Build history of the part. All positions in model axes, mm. A direction names the side the tool comes from. Coordinates: 2 decimals unless noted, no trailing zeros. Order: outer loops, then holes, each group sorted by start corner. A loop starts at its lowest first (then second) coordinate and runs counter-clockwise, first axis right, second up. Notation, with made-up numbers: M 51.5,-27.5 L 67.5,-27.5 A26 ccw 67.5,9.5 Z; hole C 35,-19.75 d8. An arc over 180 degrees is marked long. Write item = value, one per line. Start each with the question number.
Q1. Band-saw the part on B-B on x = 44.9. Write the cut outline in (y, z) (3 decimals).
Q2. 3-axis set-ups, long thin cutter, end or side, ignore diameter. For faces 4 (the face through (-47.285, 17.465, -14.711)), 5 (the face through (38, 15, -19)): which of +Z, -Z, +X, -X, +Y, -Y reach the whole face in a straight line?
Q3. Drill centre lines: probe 1 along X at (y, z) = (18.15, -13.73) (3 decimals); probe 2 along Y at (x, z) = (-82.5, -0.6) (1 decimal); probe 3 along X at (y, z) = (16, -13). Where is each one in solid material? Low to high.
Q4. Pin check, flat tips, straight feed: P1, Ø0.5, axis at y = 17.5, z = -21.5, coming from the +X side; P2, Ø7, axis at x = -32.5, z = -24.97, coming from the -Y side; P3, Ø3.5, axis at x = -82.5, y = -11, coming from the +Z side (3 decimals); P4, Ø1.1, axis at y = 17.5, z = -25.5, coming from the -X side. Stop position of each tip, or through.
Q5. Band-saw the part on C-C on z = -24.97. Write the cut outline in (x, y) (3 decimals).
Q6. Band-saw the part on A-A on y = -11. Write the cut outline in (x, z) (3 decimals).
Q7. Pull direction Z, two halves, no side cores. Call faces 1 (the face through (1, 1, -2.5)), 2 (the face through (96.5, 2, 0)), 3 (the face through (44.993, 17.465, -22.847)): released by +Z, released by -Z, zero draft, split by the parting line, or undercut.
Q8. Band-saw the part on D-D on x = -38.5. Write the cut outline in (y, z).
```python
from build123d import *

# Parameters (mm, degrees)
SKETCH1_W           = 193
SKETCH1_H           = 5
BOSS_EXTRUDE1_DEPTH = 15
BOSS_EXTRUDE2_DEPTH = 5
CUT_EXTRUDE1_REACH  = 109.344
SKETCH3_R           = 2.125
FILLET3_R           = 2
FILLET4_R           = 2
SKETCH4_R           = 2.125
CUT_EXTRUDE2_DEPTH  = 106.877004204


with BuildPart() as part:
    # Sketch1 → Boss-Extrude1 (new, symmetric)
    with BuildSketch(Plane(origin=(0, 0, 0), x_dir=(1, 0, 0), z_dir=(0, 1, 0))):
        Rectangle(SKETCH1_W, SKETCH1_H)
    extrude(amount=BOSS_EXTRUDE1_DEPTH, both=True)

    # Sketch2 → Boss-Extrude2 (add)
    with BuildSketch(Plane(origin=(0, 15, 0), x_dir=(1, 0, 0), z_dir=(0, 1, 0))):
        Polygon((-58.3, 36.2), (-58.3, 2.5), (-96.5, 2.5), (-96.5, -2.5), (96.5, -2.5), (96.5, 2.5), (57.8, 2.5), (57.8, 36.2), (19.1, 36.2), (19.1, 2.5), (-19.6, 2.5), (-19.6, 36.2), align=None)
    extrude(amount=BOSS_EXTRUDE2_DEPTH)

    # Sketch3 → Cut-Extrude1 (cut, up to next)
    with BuildSketch(Plane.XZ.offset(-15), mode=Mode.PRIVATE) as cut_extrude1_sk1:
        with Locations(Location((-45.4, -13.73, 0), (0, 0, 270))):
            Circle(SKETCH3_R)
    cut_extrude1_tool1 = extrude(cut_extrude1_sk1.sketch, amount=-CUT_EXTRUDE1_REACH, mode=Mode.PRIVATE) & part.part
    # Sketch3 → Cut-Extrude1 (cut, up to next)
    with BuildSketch(Plane.XZ.offset(-15), mode=Mode.PRIVATE) as cut_extrude1_sk2:
        with Locations(Location((-32.5, -24.97, 0), (0, 0, 270))):
            Circle(SKETCH3_R)
    cut_extrude1_tool2 = extrude(cut_extrude1_sk2.sketch, amount=-CUT_EXTRUDE1_REACH, mode=Mode.PRIVATE) & part.part
    # Sketch3 → Cut-Extrude1 (cut, up to next)
    with BuildSketch(Plane.XZ.offset(-15), mode=Mode.PRIVATE) as cut_extrude1_sk3:
        with Locations(Location((32, -13.73, 0), (0, 0, 270))):
            Circle(SKETCH3_R)
    cut_extrude1_tool3 = extrude(cut_extrude1_sk3.sketch, amount=-CUT_EXTRUDE1_REACH, mode=Mode.PRIVATE) & part.part
    # Sketch3 → Cut-Extrude1 (cut, up to next)
    with BuildSketch(Plane.XZ.offset(-15), mode=Mode.PRIVATE) as cut_extrude1_sk4:
        with Locations(Location((44.9, -24.97, 0), (0, 0, 270))):
            Circle(SKETCH3_R)
    cut_extrude1_tool4 = extrude(cut_extrude1_sk4.sketch, amount=-CUT_EXTRUDE1_REACH, mode=Mode.PRIVATE) & part.part
    add(cut_extrude1_tool1.solids().sort_by_distance((-45.4, 15, -13.73))[0], mode=Mode.SUBTRACT)
    add(cut_extrude1_tool2.solids().sort_by_distance((-32.5, 15, -24.97))[0], mode=Mode.SUBTRACT)
    add(cut_extrude1_tool3.solids().sort_by_distance((32, 15, -13.73))[0], mode=Mode.SUBTRACT)
    add(cut_extrude1_tool4.solids().sort_by_distance((44.9, 15, -24.97))[0], mode=Mode.SUBTRACT)

    # Fillet3
    fillet3_edges = [part.edges().sort_by_distance(p)[0] for p in [
        (-58.3, 17.5, -36.2),
        (-58.3, 17.5, -2.5),
        (57.8, 17.5, -2.5),
        (57.8, 17.5, -36.2),
        (19.1, 17.5, -36.2),
        (19.1, 17.5, -2.5),
        (-19.6, 17.5, -2.5),
        (-19.6, 17.5, -36.2),
    ]]
    fillet(fillet3_edges, radius=FILLET3_R)

    # Fillet4
    # the kernel refuses this fillet: 2 mm, written as the material it takes off along each edge
    with BuildSketch(Plane(origin=(21.1, 20, -34.2), x_dir=(-1, 0, 0), z_dir=(0, 0, 1))) as fillet4_piece_1:
        with BuildLine():
            CenterArc((2 - FILLET4_R, FILLET4_R), FILLET4_R, 270, 90)
            Line((2 - FILLET4_R, 0), (2, 0))
            Line((2, 0), (2, FILLET4_R))
        make_face()
    revolve(axis=Axis((21.1, 20, -34.2), (0, -1, 0)), revolution_arc=90, mode=Mode.SUBTRACT)
    with BuildSketch(Plane(origin=(-21.6, 20, -34.2), x_dir=(1, 0, 0), z_dir=(0, 0, 1))) as fillet4_piece_2:
        with BuildLine():
            CenterArc((2 - FILLET4_R, -FILLET4_R), FILLET4_R, 0, 90)
            Line((2 - FILLET4_R, 0), (2, 0))
            Line((2, 0), (2, -FILLET4_R))
        make_face()
    revolve(axis=Axis((-21.6, 20, -34.2), (0, 1, 0)), revolution_arc=90, mode=Mode.SUBTRACT)
    with BuildSketch(Plane(origin=(-56.3, 20, -34.2), x_dir=(-1, 0, 0), z_dir=(0, 0, 1))) as fillet4_piece_3:
        with BuildLine():
            CenterArc((2 - FILLET4_R, FILLET4_R), FILLET4_R, 270, 90)
            Line((2 - FILLET4_R, 0), (2, 0))
            Line((2, 0), (2, FILLET4_R))
        make_face()
    revolve(axis=Axis((-56.3, 20, -34.2), (0, -1, 0)), revolution_arc=90, mode=Mode.SUBTRACT)
    with BuildSketch(Plane(origin=(19.1, 15, -34.2), x_dir=(0, 1, 0), z_dir=(0, 0, 1)), Plane(origin=(57.8, 15, -4.5), x_dir=(0, 1, 0), z_dir=(0, 0, -1)), Plane(origin=(-19.6, 15, -4.5), x_dir=(0, 1, 0), z_dir=(0, 0, -1)), Plane(origin=(-58.3, 15, -34.2), x_dir=(0, 1, 0), z_dir=(0, 0, 1))) as fillet4_piece_4:
        with BuildLine():
            CenterArc((FILLET4_R, -FILLET4_R), FILLET4_R, 90, 90)
            Line((0, -FILLET4_R), (0, 0))
            Line((0, 0), (FILLET4_R, 0))
        make_face()
    extrude(amount=29.7, mode=Mode.SUBTRACT)
    with BuildSketch(Plane(origin=(55.8, 15, -36.2), x_dir=(0, 1, 0), z_dir=(-1, 0, 0)), Plane(origin=(-21.6, 15, -36.2), x_dir=(0, 1, 0), z_dir=(-1, 0, 0))) as fillet4_piece_5:
        with BuildLine():
            CenterArc((FILLET4_R, -FILLET4_R), FILLET4_R, 90, 90)
            Line((0, -FILLET4_R), (0, 0))
            Line((0, 0), (FILLET4_R, 0))
        make_face()
    extrude(amount=34.7, mode=Mode.SUBTRACT)
    with BuildSketch(Plane(origin=(55.8, 15, -34.2), x_dir=(1, 0, 0), z_dir=(0, 0, 1))) as fillet4_piece_6:
        with BuildLine():
            CenterArc((2 - FILLET4_R, FILLET4_R), FILLET4_R, 270, 90)
            Line((2 - FILLET4_R, 0), (2, 0))
            Line((2, 0), (2, FILLET4_R))
        make_face()
    revolve(axis=Axis((55.8, 15, -34.2), (0, 1, 0)), revolution_arc=90, mode=Mode.SUBTRACT)
    with BuildSketch(Plane(origin=(21.1, 15, -34.2), x_dir=(-1, 0, 0), z_dir=(0, 0, 1))) as fillet4_piece_7:
        with BuildLine():
            CenterArc((2 - FILLET4_R, -FILLET4_R), FILLET4_R, 0, 90)
            Line((2 - FILLET4_R, 0), (2, 0))
            Line((2, 0), (2, -FILLET4_R))
        make_face()
    revolve(axis=Axis((21.1, 15, -34.2), (0, -1, 0)), revolution_arc=90, mode=Mode.SUBTRACT)
    with BuildSketch(Plane(origin=(-17.6, 15, -4.5), x_dir=(0.5976672776328267, 0, -0.8017442392976488), z_dir=(-0.8017442392976488, 0, -0.5976672776328267))) as fillet4_piece_8_section:
        with BuildLine():
            CenterArc((2 + FILLET4_R, -FILLET4_R), FILLET4_R, 90, 90)
            Line((2, -FILLET4_R), (2, 0))
            Line((2, 0), (2 + FILLET4_R, 0))
        make_face()
    fillet4_piece_8 = revolve(axis=Axis((-17.6, 15, -4.5), (0, -1, 0)), revolution_arc=233.296989237, mode=Mode.PRIVATE)
    fillet4_piece_8 = split(fillet4_piece_8, bisect_by=Plane(origin=(-19.099877837, 15.623256941, -2.5), z_dir=(0, 0, -1)), keep=Keep.TOP, mode=Mode.PRIVATE)
    add(fillet4_piece_8, mode=Mode.SUBTRACT)
    with BuildSketch(Plane(origin=(-17.6, 20, -4.5), x_dir=(0, 0, 1), z_dir=(1, 0, 0))) as fillet4_piece_9:
        with BuildLine():
            CenterArc((2 + FILLET4_R, FILLET4_R), FILLET4_R, 180, 90)
            Line((2 + FILLET4_R, 0), (2, 0))
            Line((2, 0), (2, FILLET4_R))
        make_face()
    revolve(axis=Axis((-17.6, 20, -4.5), (0, -1, 0)), revolution_arc=90, mode=Mode.SUBTRACT)
    with BuildSketch(Plane(origin=(-60.3, 15, -4.5), x_dir=(-0.5976672776328267, 0, -0.8017442392976488), z_dir=(0.8017442392976488, 0, -0.5976672776328267))) as fillet4_piece_10_section:
        with BuildLine():
            CenterArc((2 + FILLET4_R, FILLET4_R), FILLET4_R, 180, 90)
            Line((2 + FILLET4_R, 0), (2, 0))
            Line((2, 0), (2, FILLET4_R))
        make_face()
    fillet4_piece_10 = revolve(axis=Axis((-60.3, 15, -4.5), (0, 1, 0)), revolution_arc=233.296989237, mode=Mode.PRIVATE)
    fillet4_piece_10 = split(fillet4_piece_10, bisect_by=Plane(origin=(-58.800122111, 15.623256622, -2.5), z_dir=(0, 0, -1)), keep=Keep.TOP, mode=Mode.PRIVATE)
    add(fillet4_piece_10, mode=Mode.SUBTRACT)
    with BuildSketch(Plane(origin=(-60.3, 20, -4.5), x_dir=(0, 0, 1), z_dir=(-1, 0, 0))) as fillet4_piece_11:
        with BuildLine():
            CenterArc((2 + FILLET4_R, -FILLET4_R), FILLET4_R, 90, 90)
            Line((2 + FILLET4_R, 0), (2, 0))
            Line((2, 0), (2, -FILLET4_R))
        make_face()
    revolve(axis=Axis((-60.3, 20, -4.5), (0, 1, 0)), revolution_arc=90, mode=Mode.SUBTRACT)
    with BuildSketch(Plane(origin=(17.1, 15, -4.5), x_dir=(-0.5976672776328281, 0, -0.8017442392976479), z_dir=(0.8017442392976479, 0, -0.5976672776328281))) as fillet4_piece_12_section:
        with BuildLine():
            CenterArc((2 + FILLET4_R, FILLET4_R), FILLET4_R, 180, 90)
            Line((2 + FILLET4_R, 0), (2, 0))
            Line((2, 0), (2, FILLET4_R))
        make_face()
    fillet4_piece_12 = revolve(axis=Axis((17.1, 15, -4.5), (0, 1, 0)), revolution_arc=233.296989237, mode=Mode.PRIVATE)
    fillet4_piece_12 = split(fillet4_piece_12, bisect_by=Plane(origin=(18.599877909, 15.623256541, -2.5), z_dir=(0, 0, -1)), keep=Keep.TOP, mode=Mode.PRIVATE)
    add(fillet4_piece_12, mode=Mode.SUBTRACT)
    with BuildSketch(Plane(origin=(17.1, 20, -4.5), x_dir=(0, 0, 1), z_dir=(-1, 0, 0))) as fillet4_piece_13:
        with BuildLine():
            CenterArc((2 + FILLET4_R, -FILLET4_R), FILLET4_R, 90, 90)
            Line((2 + FILLET4_R, 0), (2, 0))
            Line((2, 0), (2, -FILLET4_R))
        make_face()
    revolve(axis=Axis((17.1, 20, -4.5), (0, 1, 0)), revolution_arc=90, mode=Mode.SUBTRACT)
    with BuildSketch(Plane(origin=(59.8, 15, -4.5), x_dir=(0.5976672776328267, 0, -0.8017442392976488), z_dir=(-0.8017442392976488, 0, -0.5976672776328267))) as fillet4_piece_14_section:
        with BuildLine():
            CenterArc((2 + FILLET4_R, -FILLET4_R), FILLET4_R, 90, 90)
            Line((2, -FILLET4_R), (2, 0))
            Line((2, 0), (2 + FILLET4_R, 0))
        make_face()
    fillet4_piece_14 = revolve(axis=Axis((59.8, 15, -4.5), (0, -1, 0)), revolution_arc=233.296989237, mode=Mode.PRIVATE)
    fillet4_piece_14 = split(fillet4_piece_14, bisect_by=Plane(origin=(58.300122152, 15.623256947, -2.5), z_dir=(0, 0, -1)), keep=Keep.TOP, mode=Mode.PRIVATE)
    add(fillet4_piece_14, mode=Mode.SUBTRACT)
    with BuildSketch(Plane(origin=(59.8, 20, -4.5), x_dir=(0, 0, 1), z_dir=(1, 0, 0))) as fillet4_piece_15:
        with BuildLine():
            CenterArc((2 + FILLET4_R, FILLET4_R), FILLET4_R, 180, 90)
            Line((2 + FILLET4_R, 0), (2, 0))
            Line((2, 0), (2, FILLET4_R))
        make_face()
    revolve(axis=Axis((59.8, 20, -4.5), (0, -1, 0)), revolution_arc=90, mode=Mode.SUBTRACT)
    with BuildSketch(Plane(origin=(101.5, 20, -2.5), x_dir=(0, -1, 0), z_dir=(-1, 0, 0))) as fillet4_piece_16:
        with BuildLine():
            CenterArc((FILLET4_R, FILLET4_R), FILLET4_R, 180, 90)
            Line((0, FILLET4_R), (0, 0))
            Line((0, 0), (FILLET4_R, 0))
        make_face()
    extrude(amount=41.7, mode=Mode.SUBTRACT)
    with BuildSketch(Plane(origin=(-19.6, 20, -4.5), x_dir=(0, -1, 0), z_dir=(0, 0, -1)), Plane(origin=(-58.3, 20, -34.2), x_dir=(0, -1, 0), z_dir=(0, 0, 1)), Plane(origin=(57.8, 20, -4.5), x_dir=(0, -1, 0), z_dir=(0, 0, -1)), Plane(origin=(19.1, 20, -34.2), x_dir=(0, -1, 0), z_dir=(0, 0, 1))) as fillet4_piece_17:
        with BuildLine():
            CenterArc((FILLET4_R, FILLET4_R), FILLET4_R, 180, 90)
            Line((0, FILLET4_R), (0, 0))
            Line((0, 0), (FILLET4_R, 0))
        make_face()
    extrude(amount=29.7, mode=Mode.SUBTRACT)
    with BuildSketch(Plane(origin=(-60.3, 20, -2.5), x_dir=(0, -1, 0), z_dir=(-1, 0, 0))) as fillet4_piece_18:
        with BuildLine():
            CenterArc((FILLET4_R, FILLET4_R), FILLET4_R, 180, 90)
            Line((0, FILLET4_R), (0, 0))
            Line((0, 0), (FILLET4_R, 0))
        make_face()
    extrude(amount=41.2, mode=Mode.SUBTRACT)
    with BuildSketch(Plane(origin=(17.1, 20, -2.5), x_dir=(0, -1, 0), z_dir=(-1, 0, 0)), Plane(origin=(-21.6, 20, -36.2), x_dir=(0, -1, 0), z_dir=(-1, 0, 0)), Plane(origin=(55.8, 20, -36.2), x_dir=(0, -1, 0), z_dir=(-1, 0, 0))) as fillet4_piece_19:
        with BuildLine():
            CenterArc((FILLET4_R, FILLET4_R), FILLET4_R, 180, 90)
            Line((0, FILLET4_R), (0, 0))
            Line((0, 0), (FILLET4_R, 0))
        make_face()
    extrude(amount=34.7, mode=Mode.SUBTRACT)
    with BuildSketch(Plane(origin=(-21.6, 15, -34.2), x_dir=(1, 0, 0), z_dir=(0, 0, 1))) as fillet4_piece_20:
        with BuildLine():
            CenterArc((2 - FILLET4_R, FILLET4_R), FILLET4_R, 270, 90)
            Line((2 - FILLET4_R, 0), (2, 0))
            Line((2, 0), (2, FILLET4_R))
        make_face()
    revolve(axis=Axis((-21.6, 15, -34.2), (0, 1, 0)), revolution_arc=90, mode=Mode.SUBTRACT)
    with BuildSketch(Plane(origin=(-56.3, 15, -34.2), x_dir=(-1, 0, 0), z_dir=(0, 0, 1))) as fillet4_piece_21:
        with BuildLine():
            CenterArc((2 - FILLET4_R, -FILLET4_R), FILLET4_R, 0, 90)
            Line((2 - FILLET4_R, 0), (2, 0))
            Line((2, 0), (2, -FILLET4_R))
        make_face()
    revolve(axis=Axis((-56.3, 15, -34.2), (0, -1, 0)), revolution_arc=90, mode=Mode.SUBTRACT)
    with BuildSketch(Plane(origin=(55.8, 20, -34.2), x_dir=(1, 0, 0), z_dir=(0, 0, 1))) as fillet4_piece_22:
        with BuildLine():
            CenterArc((2 - FILLET4_R, -FILLET4_R), FILLET4_R, 0, 90)
            Line((2 - FILLET4_R, 0), (2, 0))
            Line((2, 0), (2, -FILLET4_R))
        make_face()
    revolve(axis=Axis((55.8, 20, -34.2), (0, 1, 0)), revolution_arc=90, mode=Mode.SUBTRACT)

    # Sketch4 → Cut-Extrude2 (cut, through all)
    with BuildSketch(Plane.XY.offset(2.5)):
        with Locations((-82.5, 9)):
            Circle(SKETCH4_R)
        with Locations((-82.5, -11)):
            Circle(SKETCH4_R)
    extrude(amount=-CUT_EXTRUDE2_DEPTH, mode=Mode.SUBTRACT)


solid = part.part
```
Recorded:
q1.outline = M -15,-2.5 L 15,-2.5 L 15,-22.845 L 20,-22.845 L 20,2.5 L -15,2.5 Z; M 15,-34.2 A2 ccw 17,-36.2 L 18,-36.2 A2 ccw 20,-34.2 L 20,-27.095 L 15,-27.095 Z
q2.face_4 = +Y, -Y
q2.face_5 = -Z, +X, -X, -Y
q3.probe_1 = -58.294 to -47.525, -43.275 to -19.606, 19.106 to 29.875, 34.125 to 57.794
q3.probe_2 = -15 to -13.1, -8.9 to 6.9, 11.1 to 20
q3.probe_3 = -58.03 to -47.4, -43.4 to -19.87, 19.37 to 30, 34 to 57.53
q4.P1 = 57.8
q4.P2 = 15
q4.P3 = through
q4.P4 = -58.3
q5.outline = M -58.3,17 A2 ccw -56.3,15 L -34.625,15 L -34.625,20 L -56.3,20 A2 ccw -58.3,18 Z; M -30.375,15 L -21.6,15 A2 ccw -19.6,17 L -19.6,18 A2 ccw -21.6,20 L -30.375,20 Z; M 19.1,17 A2 ccw 21.1,15 L 42.775,15 L 42.775,20 L 21.1,20 A2 ccw 19.1,18 Z; M 47.025,15 L 55.8,15 A2 ccw 57.8,17 L 57.8,18 A2 ccw 55.8,20 L 47.025,20 Z
q6.outline = M -96.5,-2.5 L -84.625,-2.5 L -84.625,2.5 L -96.5,2.5 Z; M -80.375,-2.5 L 96.5,-2.5 L 96.5,2.5 L -80.375,2.5 Z
q7.face_1 = released by -Z
q7.face_2 = zero draft
q7.face_3 = undercut
q8.outline = M -15,-2.5 L 15,-2.5 L 15,-34.2 A2 ccw 17,-36.2 L 18,-36.2 A2 ccw 20,-34.2 L 20,2.5 L -15,2.5 Z
